Could you check a few things on this drawing? It's one solid part, dimensions in mm from its lowest x, y, z. Give positions to 0.01 mm unless a question says otherwise; leave off trailing zeros. Loops run counter-clockwise (first coordinate to the right, second up) from the corner with the lowest first, then second, coordinate; pieces in that order, holes last. Notation, with made-up numbers: M 77.25,16 L 96.25,16 A14 ccw 96.25,29 Z; hole C 44.25,-21 d11. An arc over 180 degrees is marked long. Answer in a Markdown table with one row per item. Add a question column.
1. Thinking about a two-plate mould opening in X: for the marked faces 1 and 2, which applies, released by +X, released by -X, zero draft, split by the parting line, or undercut?
2. I need wall thicknesses on line 1 along X through (y, z) = (5.95, 0.2) (1 decimal); line 2 along Y through (x, z) = (7.7, 0.25); line 3 along X through (y, z) = (7.25, 0.6). Which ranges of each line are inside material? Lowest first, please. Write a range as from..to.
3. If we section it at D-D on y = 5.95: Count the separate pieces of the cut face and the enclosed holes in it.
4. If we section it at B-B on y = 7.7: List the corners of the cut face in (x, z) for me.
5. If we section it at A-A on x = 7.7: List the corners of the cut face in (y, z) for me.
6. If we section it at C-C on z = 0.2: List the corners of the cut face in (x, y) for me.
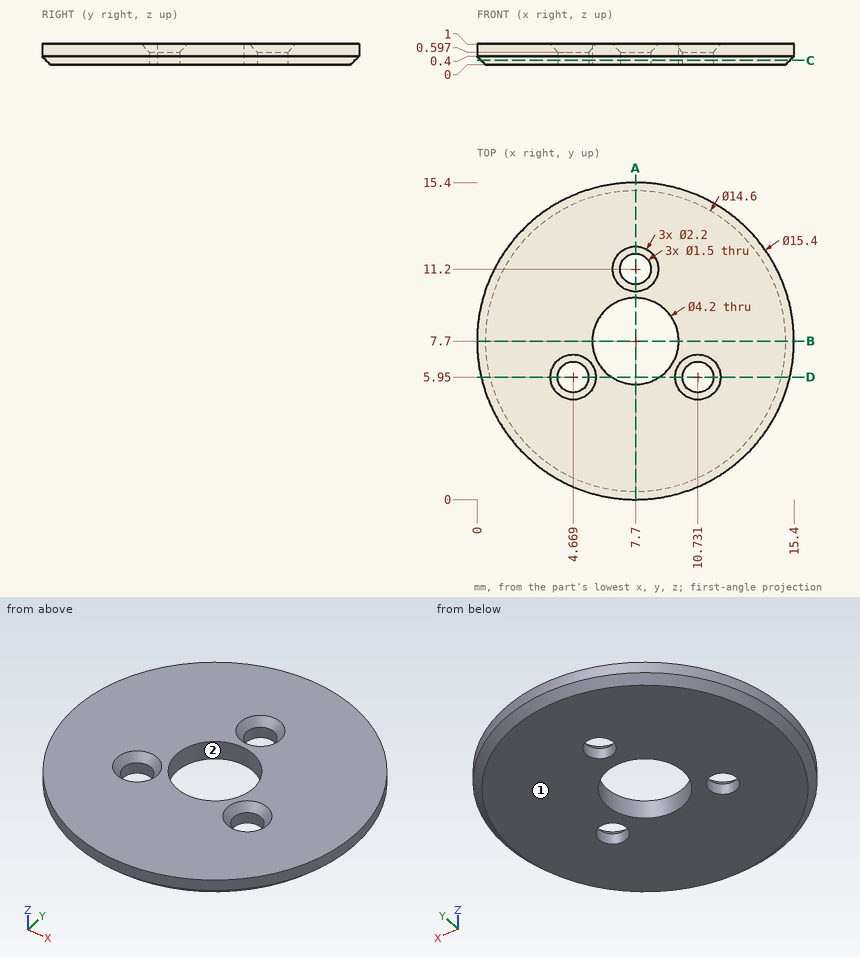
Results:
| question | item | result |
|---|---|---|
| 1 | face 1 | zero draft |
| 1 | face 2 | undercut |
| 2 | line 1 | 0.4..3.9, 5.4..6.5, 8.9..10, 11.5..15 |
| 2 | line 2 | 0.15..5.6, 9.8..10.45, 11.95..15.25 |
| 2 | line 3 | 0.01..5.65, 9.75..15.39 |
| 3 | separate pieces | 4 |
| 3 | enclosed holes | 0 |
| 4 | outline | M 0,0.4 L 0.4,0 L 5.6,0 L 5.6,1 L 0,1 Z; M 9.8,0 L 15,0 L 15.4,0.4 L 15.4,1 L 9.8,1 Z |
| 5 | outline | M 0,0.4 L 0.4,0 L 5.6,0 L 5.6,1 L 0,1 Z; M 9.8,0 L 10.45,0 L 10.45,0.6 L 10.1,1 L 9.8,1 Z; M 11.95,0 L 15,0 L 15.4,0.4 L 15.4,1 L 12.3,1 L 11.95,0.6 Z |
| 6 | outline | C 7.7,7.7 d15; hole C 4.67,5.95 d1.5; hole C 7.7,7.7 d4.2; hole C 7.7,11.2 d1.5; hole C 10.73,5.95 d1.5 |
